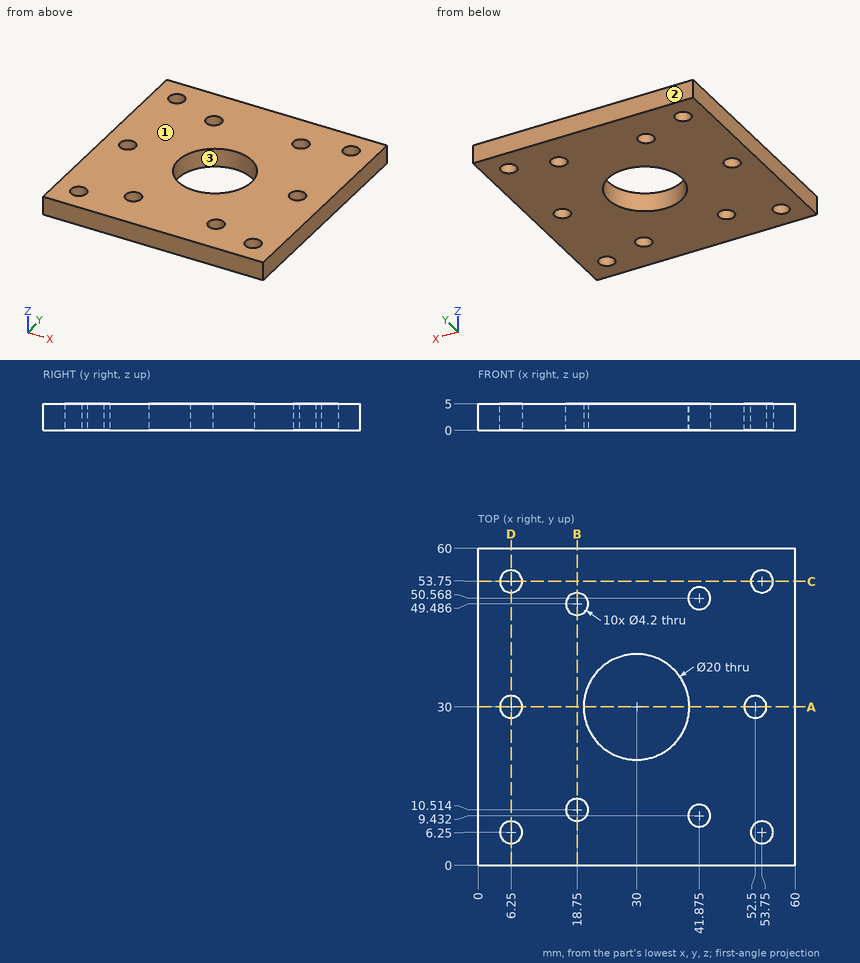
Answer from the drawing. Dimensions are ordinates in mm from the lowest x, y and z of the part. Round coordinates to 2 decimals unless told otherwise and drop trailing zeros. Order: outer loops, then holes, each group sorted by start corner. A loop starts at its lowest first (then second) coordinate and runs counter-clockwise, first axis right, second up.
1) The part is cut by section B-B on x = 18.75. Write down the section's boundary in (y, z) (1 decimal), plus the area to 3 significant figures.
2) The part is cut by section D-D on x = 6.25. Write down the section's boundary in (y, z).
3) The part is cut by section A-A on y = 30. Write down the section's boundary in (x, z), plus the area to 3 significant figures.
4) Flat-ended cylindrical pins translate along their axes: pin 1 (5.5 mm diameter, centred on x = 53.75, y = 53.75, fed in from -Z); pin 2 (2.5 mm diameter, centred on x = 52.5, y = 30, fed in from +Z). Find the tip coordinate at first contact, or state that the pin passes through.
5) Straight lines are drawn through the part: L1, parallel to X at y = 6.25, z = 3.3; L2, parallel to Y at x = 6, z = 3.25 (1 decimal); L3, parallel to Y at x = 42, z = 4.15 (1 decimal). For each, find the intervals that lie inside material, in ascending order.
6) The part is cut by section C-C on y = 53.75. Write down the section's boundary in (x, z), plus the area to 3 significant figures.
7) The mould has two halves that part along Y. Classify the marked faces 1, 2 and 3: released by +Y, released by -Y, zero draft, split by the parting line, or undercut.
Resolved:
1. outline: (0, 0) - (8.4, 0) - (8.4, 5) - (0, 5) - close; (12.6, 0) - (47.4, 0) - (47.4, 5) - (12.6, 5) - close; (51.6, 0) - (60, 0) - (60, 5) - (51.6, 5) - close
1. area: 258 mm2
2. outline: (0, 0) - (4.15, 0) - (4.15, 5) - (0, 5) - close; (8.35, 0) - (27.9, 0) - (27.9, 5) - (8.35, 5) - close; (32.1, 0) - (51.65, 0) - (51.65, 5) - (32.1, 5) - close; (55.85, 0) - (60, 0) - (60, 5) - (55.85, 5) - close
3. outline: (0, 0) - (4.15, 0) - (4.15, 5) - (0, 5) - close; (8.35, 0) - (20, 0) - (20, 5) - (8.35, 5) - close; (40, 0) - (50.4, 0) - (50.4, 5) - (40, 5) - close; (54.6, 0) - (60, 0) - (60, 5) - (54.6, 5) - close
3. area: 158 mm2
4. pin 1: stops at z = 0
4. pin 2: passes through
5. L1: x = 0 to 4.15, 8.35 to 51.65, 55.85 to 60
5. L2: y = 0 to 4.2, 8.3 to 27.9, 32.1 to 51.7, 55.8 to 60
5. L3: y = 0 to 7.3, 11.5 to 48.5, 52.7 to 60
6. outline: (0, 0) - (4.15, 0) - (4.15, 5) - (0, 5) - close; (8.35, 0) - (51.65, 0) - (51.65, 5) - (8.35, 5) - close; (55.85, 0) - (60, 0) - (60, 5) - (55.85, 5) - close
6. area: 258 mm2
7. face 1: zero draft
7. face 2: released by +Y
7. face 3: undercut
